Can you work these out from the model? Positions are in its coordinate system, mm. Face numbers are marked on the shaded views. Coordinates: 2 decimals unless noted, no trailing zeros. Loops run counter-clockwise (first coordinate to the right, second up) from the corner with the lowest first, then second, coordinate; pieces in that order, holes last.
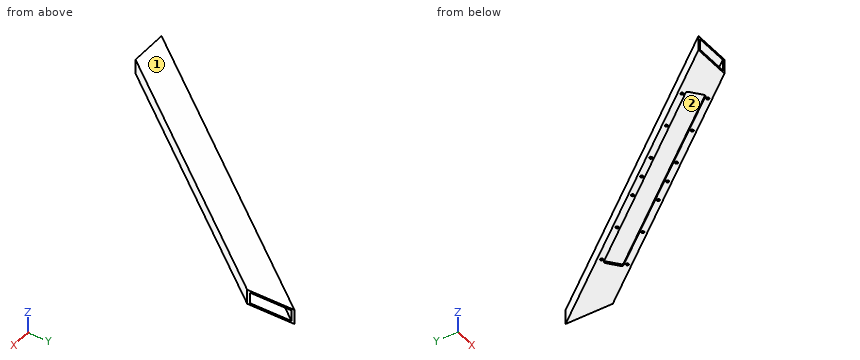
```python
from build123d import *

# Parameters (mm, degrees)
BOSS_EXTRUDE1_DEPTH = 25.4
SHELL1_T            = -3.175
CUT_EXTRUDE1_START  = -7.62
SKETCH2_R           = 2.38125
CUT_EXTRUDE1_DEPTH  = 644.433085393
FILLET1_R           = 3.175


with BuildPart() as part:
    # Sketch1 → Boss-Extrude1 (new body)
    with BuildSketch(Plane.XY):
        Polygon((0, 0), (406.4, 508), (406.4, 426.680322185), (65.055742252, 0), align=None)
    extrude(amount=BOSS_EXTRUDE1_DEPTH)

    # Shell1
    shell1_openings = [part.faces().sort_by_distance(p)[0] for p in [
        (406.4, 467.340161092, 12.7),
        (32.527871126, 0, 12.7),
    ]]
    offset(amount=SHELL1_T, openings=shell1_openings, kind=Kind.INTERSECTION)

    # Sketch2 → Cut-Extrude1 (cut, through all)
    with BuildSketch(Plane.XY.offset(25.4).offset(CUT_EXTRUDE1_START)):
        with Locations((68.427533771, 75.369457487)):
            Circle(SKETCH2_R)
        with Locations((116.029296395, 134.871660767)):
            Circle(SKETCH2_R)
        with Locations((163.631059019, 194.373864047)):
            Circle(SKETCH2_R)
        with Locations((193.382160659, 170.572982735)):
            Circle(SKETCH2_R)
        with Locations((145.780398035, 111.070779455)):
            Circle(SKETCH2_R)
        with Locations((98.178635411, 51.568576176)):
            Circle(SKETCH2_R)
        with Locations((344.121075633, 358.996626453)):
            Circle(SKETCH2_R)
        with Locations((296.51931301, 299.494423174)):
            Circle(SKETCH2_R)
        with Locations((248.917550386, 239.992219894)):
            Circle(SKETCH2_R)
        with Locations((219.166448746, 263.793101206)):
            Circle(SKETCH2_R)
        with Locations((266.76821137, 323.295304486)):
            Circle(SKETCH2_R)
        with Locations((314.369973994, 382.797507765)):
            Circle(SKETCH2_R)
        with Locations((191.398753883, 229.083482626)):
            Circle(SKETCH2_R)
        with Locations((221.149855522, 205.282601314)):
            Circle(SKETCH2_R)
        Polygon((90.740860001, 49.386828722), (344.616927327, 366.73191288), (321.807749404, 384.979255219), (67.931682077, 67.634171061), align=None)
    extrude(amount=-CUT_EXTRUDE1_DEPTH, mode=Mode.SUBTRACT)

    # Fillet1
    fillet1_edges = [part.edges().sort_by_distance(p)[0] for p in [
        (90.740860001, 49.386828722, 1.5875),
        (67.931682077, 67.634171061, 1.5875),
        (321.807749404, 384.979255219, 1.5875),
        (344.616927327, 366.73191288, 1.5875),
    ]]
    fillet(fillet1_edges, radius=FILLET1_R)


solid = part.part
```
Item 1: I'm going to push flat-ended pins straight in: P1, Ø3, axis at x = 314.37, y = 382.8, coming from the -Z side (3 decimals); P2, Ø6, axis at x = 192, z = 8.5, coming from the -Y side; P3, Ø10, axis at x = 226, z = 15, coming from the -Y side. Where does each tip first touch, or does it pass through?
Results are:
P1: stops at z = 22.225
P2: stops at y = 154.93
P3: stops at y = 194.93
Item 2: Suppose I cut it at B-B, the plane y = 184. Please give me the cut outline in (x, z) (3 decimals), plus the area to 3 significant figures.
Results are:
outline: (147.2, 0) - (161.024, 0) - (161.024, 3.175) - (151.266, 3.175) - (151.266, 22.225) - (208.19, 22.225) - (208.19, 3.175) - (198.431, 3.175) - (198.431, 0) - (212.256, 0) - (212.256, 25.4) - (147.2, 25.4) - close
area: 449 mm2
Item 3: I need wall thicknesses on line 1 along Z through (x, y) = (213.5, 214.5) (3 decimals); line 2 along Y through (x, z) = (145, 5); line 3 along X through (y, z) = (56.5, 17.75). Which ranges of each line are inside material? Lowest first, please.
Results are:
line 1: z = 22.225 to 25.4
line 2: y = 99.93 to 105.01, 176.17 to 181.25
line 3: x = 45.2 to 49.27, 106.19 to 110.26
Item 4: We'd pull the mould along Y, two halves only. Please class the marked faces 1 and 2: +Y half, -Y half, draft (parallel to the pull), parting line (faces both ways), or undercut.
Results are:
face 1: draft
face 2: undercut
Item 5: Suppose I cut it at C-C, the plane y = 462.5. Please give me the cut outline in (x, z) (3 decimals), plus the area to 3 significant figures.
Results are:
outline: (370, 0) - (406.4, 0) - (406.4, 3.175) - (374.066, 3.175) - (374.066, 22.225) - (406.4, 22.225) - (406.4, 25.4) - (370, 25.4) - close
area: 309 mm2
Item 6: Suppose I cut it at A-A, the plane z = 11.25. Please give me the cut outline in (x, y).
Results are:
outline: (0, 0) - (4.07, 0) - (406.4, 502.92) - (406.4, 508) - close; (60.99, 0) - (65.06, 0) - (406.4, 426.68) - (406.4, 431.76) - close
